Geometry check sheet. Reference: drawing and pictorial views, mm from the part's lowest x, y, z. Coordinates: 2 decimals unless noted, no trailing zeros. Loops run counter-clockwise (first coordinate to the right, second up) from the corner with the lowest first, then second, coordinate; pieces in that order, holes last. Notation, with made-up numbers: (-18.5, 13.25) -> (9.5, 13.25) arc R36 cw to (9.5, 47.25) -> close; hole circle Ø7 at (86, -39). An arc over 180 degrees is marked (long way). Answer as a JSON object with one key per item and string values. Group by question number.
Q1. Cross-section at A-A on z = 30.5. Record the boundary of the cut face in (x, y).
Q2. Cross-section at C-C on y = 1. Give the number of separate pieces and of enclosed holes in the cut face, and give its area (3 significant figures).
Q3. Cross-section at D-D on x = 57. Record the boundary of the cut face in (y, z).
Q4. Gauge pin test, flat ends, axial feed: pin 1 Ø4.5 at (x, z) = (52.77, 38.63) entering from -Y; pin 2 Ø1.7 at (x, z) = (8.23, 38.63) entering from -Y; pin 3 Ø1.5 at (y, z) = (2.5, 51) entering from +X; pin 4 Ø1.5 at (x, y) = (6.5, 1.5) entering from -Z. Record the tip position at first contact, or that the pin passes through.
Q5. Scan lines: L1, parallel to Z at x = 31, y = 0.6; L2, parallel to X at y = 0.85, z = 42.5 (1 decimal); L3, parallel to X at y = 0.35, z = 31.5 (1 decimal). Record each from-to range of solid material in increasing order.
Q6. Cross-section at B-B on x = 30.5. Record the boundary of the cut face in (y, z).
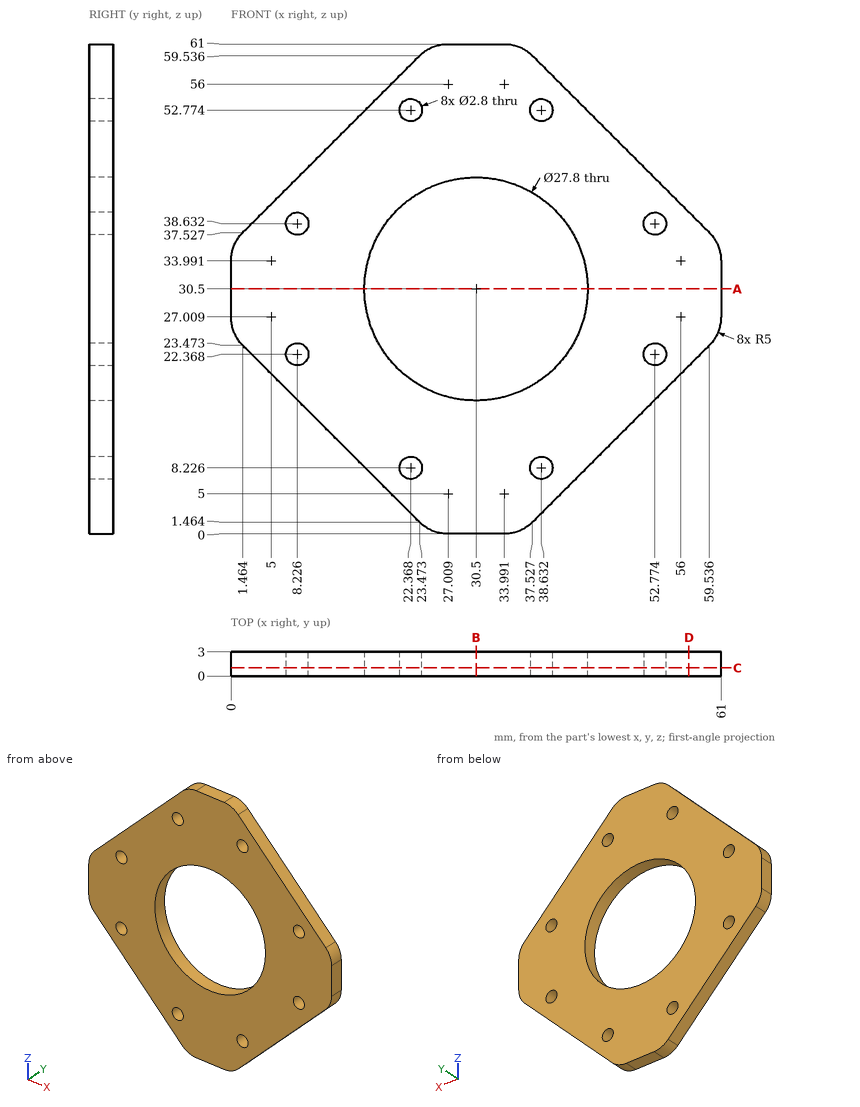
Computed values:
{
 "1": {"outline": "(0, 0) -> (16.6, 0) -> (16.6, 3) -> (0, 3) -> close; (44.4, 0) -> (61, 0) -> (61, 3) -> (44.4, 3) -> close"},
 "2": {"separate pieces": "1", "enclosed holes": "9", "area": "1,820 mm²"},
 "3": {"outline": "(0, 20.94) -> (3, 20.94) -> (3, 40.06) -> (0, 40.06) -> close"},
 "4": {"pin 1": "stops at y = 0", "pin 2": "passes through", "pin 3": "stops at x = 46.81", "pin 4": "stops at z = 17.69"},
 "5": {"L1": "z = 0 to 16.61, 44.39 to 61", "L2": "x = 6.4 to 23.5, 37.5 to 54.6", "L3": "x = 0 to 16.6, 44.4 to 61"},
 "6": {"outline": "(0, 0) -> (3, 0) -> (3, 16.6) -> (0, 16.6) -> close; (0, 44.4) -> (3, 44.4) -> (3, 61) -> (0, 61) -> close"}
}
